Here's how the part is built. I have some questions about the finished solid (model axes, mm). Coordinates: 2 decimals unless noted, no trailing zeros. Write each loop counter-clockwise with the first axis right and the second up, starting at its lowest first coordinate (ties: lowest second). Pieces come first, ordered by that corner, then holes. Notation, with made-up numbers: M 58.25,-24.75 L 106.25,-24.75 A19 cw 106.25,-8.75 Z; hole C 72.5,83 d4. An arc over 180 degrees is marked long. Use one line per item in the form item = value. Start each with the question number.
1. I want a section at C-C, the plane x = 33. List the corners of the cut face in (y, z) for me.
2. I want a section at B-B, the plane y = -33.5. List the corners of the cut face in (x, z) for me.
3. Please list where these lines run through material, in increasing order: line 1 along Y through (x, z) = (-4, 407); line 2 along X through (y, z) = (-19, 470); line 3 along Y through (x, z) = (17.5, -44). Write a range as [from, to].
4. I want a section at A-A, the plane z = -587.5. List the corners of the cut face in (x, y) for me, plus the area to 3 significant figures.
5. I'm going to push flat-ended pins straight in: pin 1 Ø5 at (x, z) = (-35, 713) entering from +Y; pin 2 Ø5 at (x, z) = (17.5, -479) entering from -Y; pin 3 Ø3 at (y, z) = (-43.5, 335.5) entering from +X. Where does each tip first touch, or does it pass through?
from build123d import *

# Parameters (mm, degrees)
SKETCH1_R           = 7.5
BOSS_EXTRUDE1_DEPTH = 250
SCALE1_SCALE        = 10
SCALE2_SCALE        = 0.75


with BuildPart() as part:
    # Sketch1 → Boss-Extrude1 (new body)
    with BuildSketch(Plane.XY):
        Circle(SKETCH1_R)
    extrude(amount=BOSS_EXTRUDE1_DEPTH)


with BuildPart() as part_1:
    # Scale1: scaled about (0, 0, 125)
    add(part.part.scale(SCALE1_SCALE).moved(Location((0, 0, -1125))))


with BuildPart() as part_2:
    # Scale2: scaled about (0, 0, 0)
    add(part_1.part.scale(SCALE2_SCALE))


solid = part_2.part
Answer list:
q1.outline = M -45.55,-843.75 L 45.55,-843.75 L 45.55,1031.25 L -45.55,1031.25 Z
q2.outline = M -45.19,-843.75 L 45.19,-843.75 L 45.19,1031.25 L -45.19,1031.25 Z
q3.line_1 = [-56.11, 56.11]
q3.line_2 = [-52.94, 52.94]
q3.line_3 = [-53.46, 53.46]
q4.outline = C 0,0 d112.5
q4.area = 9,940 mm²
q5.pin_1 = 45.91
q5.pin_2 = -54.21
q5.pin_3 = 37.42
